from build123d import *

# Parameters (mm, degrees)
SKETCH1_W           = 50.8
SKETCH1_H           = 25.4
SKETCH1_W_2         = 46.8
SKETCH1_H_2         = 21.4
BOSS_EXTRUDE1_DEPTH = 50
SKETCH2_W           = 21.4
SKETCH2_H           = 4
CUT_EXTRUDE1_DEPTH  = 76.669016116
LPATTERN1_COUNT     = 6
LPATTERN1_PITCH     = 10
LPATTERN1_COL_COUNT = 6
LPATTERN1_COL_PITCH = 10


with BuildPart() as part:
    # Sketch1 → Boss-Extrude1 (new, symmetric)
    with BuildSketch(Plane(origin=(0, 0, 0), x_dir=(1, 0, 0), z_dir=(0, 1, 0))):
        with Locations((25.4, 12.7)):
            Rectangle(SKETCH1_W, SKETCH1_H)
        with Locations((25.4, 12.7)):
            Rectangle(SKETCH1_W_2, SKETCH1_H_2, mode=Mode.SUBTRACT)
    extrude(amount=BOSS_EXTRUDE1_DEPTH, both=True)

    # Sketch2 → Cut-Extrude1 (cut, through all)
    with BuildSketch(Plane(origin=(50.8, 0, 0), x_dir=(0, 0, -1), z_dir=(1, 0, 0))):
        with Locations((12.7, 0)):
            Rectangle(SKETCH2_W, SKETCH2_H)
    cut_extrude1 = extrude(amount=-CUT_EXTRUDE1_DEPTH, mode=Mode.SUBTRACT)

    # LPattern1: Cut-Extrude1 ×6
    with Locations(*[(0, -i * LPATTERN1_PITCH, 0) for i in range(1, LPATTERN1_COUNT)]):
        add(cut_extrude1, mode=Mode.SUBTRACT)

    # LPattern1 col: Cut-Extrude1 ×6
    with Locations(*[(0, i * LPATTERN1_COL_PITCH, 0) for i in range(1, LPATTERN1_COL_COUNT)]):
        add(cut_extrude1, mode=Mode.SUBTRACT)


solid = part.part
Geometry: final body of the model. Coordinates: model frame, mm. A direction names the side the tool comes from. Round coordinates to 2 decimals unless told otherwise and drop trailing zeros. Write each loop counter-clockwise with the first axis right and the second up, starting at its lowest first coordinate (ties: lowest second). Pieces come first, ordered by that corner, then holes. Notation, with made-up numbers: M -30.5,85 L -11.5,85 A18 ccw -11.5,90 Z; hole C 7.5,-9.5 d5. An arc over 180 degrees is marked long. Write item = value, one per line.
Item 1: Section query A-A on y = 41. Return loops of the section in (x, z).
Findings:
outline = M 0,-25.4 L 50.8,-25.4 L 50.8,-23.4 L 0,-23.4 Z; M 0,-2 L 50.8,-2 L 50.8,0 L 0,0 Z
Item 2: Section query C-C on z = -11.25. State how many separate pieces and enclosed holes the cut face has, then the cut area to 3 significant figures.
Findings:
separate_pieces = 20
enclosed_holes = 0
area = 240 mm^2
Item 3: Material intervals for line 1 along X through (y, z) = (5.5, -22.25); line 2 along Z through (x, y) = (22, -35), sorted ascending. Write a range as [from, to].
Findings:
line_1 = [0, 2], [48.8, 50.8]
line_2 = [-25.4, -23.4], [-2, 0]
Item 4: Pin query (flat end, axial travel): P1, Ø1.6, axis at x = 1, z = -17.5, coming from the +Y side; P2, Ø5, axis at y = 31.5, z = -11.5, coming from the -X side; P3, Ø1, axis at x = 49.5, z = -10, coming from the -Y side; P4, Ø12, axis at x = 31, z = -16.5, coming from the +Y side. Return the tip coordinate at first contact, or that it passes through.
Findings:
P1 = 48
P2 = 0
P3 = -48
P4 = through
Item 5: Access query for faces 1 (the face through (1, -48, -13)), 2 (the face through (2, -25, -13)), 3 (the face through (50.8, 1, -24)), 4 (the face through (1, 38, -13)). Directions: +Z, -Z, +X, -X, +Y, -Y. A direction counts if a zero-diameter tool reaches every point of the face in a straight line with its end or side. Return the directions, or none.
Findings:
face_1 = +X, -X, -Y
face_2 = +Y, -Y
face_3 = +Z, -Z, +X, +Y, -Y
face_4 = +X, -X
Item 6: Pull-direction query (Z, two-part tool) for faces 5 (the face through (2, 25, -13)), 6 (the face through (25, -50, -24)); classes: pulls with the +Z half, pulls with the -Z half, needs draft (parallel to the pull), parting line crosses it, or undercut.
Findings:
face_5 = undercut
face_6 = needs draft
Item 7: Section query B-B on x = 9.5. Return loops of the section in (y, z), then the cut area to 3 significant figures.
Findings:
outline = M -50,-25.4 L 50,-25.4 L 50,-23.4 L -50,-23.4 Z; M -50,-2 L 50,-2 L 50,0 L -50,0 Z
area = 400 mm^2
